from build123d import *

# Parameters (mm, degrees)
F0_R      = 38.1
F1_DEPTH  = 30.48
F2_W      = 45.819147911
F2_H      = 7.0118308067
F3_DEPTH  = 2.54
F4_T      = -2.54
F8_DEPTH  = 9.906
F10_DEPTH = 5.08


with BuildPart() as f1:
    # F0 (on Top) → F1 (new body)
    with BuildSketch(Plane.XY):
        Circle(F0_R)
    extrude(amount=F1_DEPTH)

    # F2 (on face) → F3 (join)
    with BuildSketch(Plane.XY.offset(30.48)):
        with Locations((0.8893240733, -19.5669056848)):
            Rectangle(F2_W, F2_H)
    extrude(amount=F3_DEPTH)

    # F4 (hollow: no face is removed)
    offset(amount=F4_T, kind=Kind.INTERSECTION, mode=Mode.SUBTRACT)

    # F7 (on face) → F8 (cut)
    with BuildSketch(Plane.XY.offset(30.48)):
        Polygon((-15.4119321378, -12.1194338849), (-14.841485885, -15.7707315361), (5.0025711535, -15.7707315361), (6.1164895305, -14.8400934836), (6.1164895305, -11.340892916), (6.3189007342, -9.2710563913), (6.0210963711, -6.8141715601), (6.0048130108, -5.5709355934), (5.6325580226, -4.6775222713), (6.0792639852, -3.5607567247), (6.0792639852, -2.0221695727), (5.7286338997, -1.0273779467), (9.9040070724, 0.4442985472), (11.7219447857, 2.5462731296), (11.7219447857, 4.9659329975), (15.7423027558, 7.0877885023), (22.1039241878, 10.3067904288), (25.4188793848, 10.3067904288), (29.9926726737, 12.4215105659), (30.7439389297, 15.0509480497), (29.6866364668, 17.4833167877), (25.6525882866, 18.8981650481), (18.5155458163, 17.708657504), (16.6474783241, 16.844945549), (9.1134678884, 13.3615516624), (7.5662216179, 11.7286253879), (1.8378060551, 10.445210726), (1.149144816, 10.8521465371), (3.3716449027, 11.5721119727), (5.3750247236, 13.2937669913), (5.9697784957, 15.1093309904), (5.5432569709, 17.361162805), (5.2361546324, 17.7185181528), (2.1184887737, 17.7185181528), (1.3361625606, 21.336780861), (1.3361625606, 23.9771343768), (0, 26.2263249606), (0, 27.1613527107), (-3.5394631901, 30.5318216514), (-5.2709043957, 31.7105762661), (-8.7543707341, 32.132551074), (-11.3128684461, 31.4410664141), (-14.5628526807, 30.542133376), (-16.7756080627, 28.8825668395), (-19.0620572539, 25.78573856), (-20.3636531951, 22.1986565316), (-20.7315385342, 18.6494737864), (-19.479425624, 13.39059975), (-15.4119321378, 10.9802337791), (-19.0177896293, 7.0877885023), (-19.0177896293, 0.4442985472), (-15.4119321378, -3.7730513141), (-16.0732436925, -8.2028741017), align=None)
    extrude(amount=-F8_DEPTH, mode=Mode.SUBTRACT)

    # F9 (on face) → F10 (join)
    with BuildSketch(Plane.XY.offset(30.48)):
        Polygon((9.2707704753, 15.7535430044), (10.2326864312, 16.7216230184), (-7.1297219356, 16.7216230184), (-13.6908106506, 14.8423165083), (-17.4043960869, 9.4877332449), (-19.9085921049, 6.8410946988), (-19.9085921049, 1.7150167664), (-19.6581706405, -3.6766524427), (-15.2726136148, -5.7415137999), (-13.1471836939, -2.1741164383), (-7.5955540778, 6.8410946988), (4.2351128765, 10.4722213), (9.2707704753, 14.7913218218), align=None)
        Polygon((3.8815487642, 1.0813763365), (6.6431248561, 0.6791502237), (9.9622569978, 2.7536081616), (11.7555428296, 4.9633402377), (15.3087614144, 6.8410946988), (21.8024684188, 8.8341752525), (30.4993893951, 12.0195187628), (30.8451298624, 16.7216230184), (27.3877009749, 19.3492695689), (19.6581706405, 19.6126438677), (12.7007676991, 15.7535430044), (10.8933802694, 14.2285590991), (9.2707704753, 12.8604179814), (2.2486662492, 8.0840246186), (1.4972069766, 4.3447160861), align=None)
    extrude(amount=F10_DEPTH)


solid = f1.part
The model under review builds one solid part; all positions refer to its coordinate system, in mm. A direction names the side the tool comes from. Round coordinates to 2 decimals unless told otherwise and drop trailing zeros. Write each loop counter-clockwise with the first axis right and the second up, starting at its lowest first coordinate (ties: lowest second). Pieces come first, ordered by that corner, then holes. Notation, with made-up numbers: (-15, 37) - (36, 37) arc R33 ccw to (36, 69) - close; hole circle Ø5 at (31.25, 54.5). An arc over 180 degrees is marked (long way). One line per item, written item: value. Start each with the question number.
1. The part is to be moulded in two halves that separate along Y. For faces 5 (the face through (1, -23.073, 32)), 6 (the face through (-15.522, 12.203, 32.984)), 7 (the face through (2.7, 2.7, 33)), say which applies: released by +Y, released by -Y, zero draft, split by the parting line, or undercut.
2. Machinability: for faces 1 (the face through (10.846, 3.843, 32.984)), 2 (the face through (-22.02, -20, 32)), 3 (the face through (-4.39, 31.11, 29.23)), 4 (the face through (2.245, 11.207, 29.228)), which of the approach directions +Z, -Z, +X, -X, +Y, -Y give a long, thin tool a straight path to every point of the face, cutting with its end or side? Answer none if there is none.
3. Clearance check with flat-ended pins moving along their axes: P1, Ø2, axis at y = -19, z = 26.5, coming from the +X side; P2, Ø8, axis at x = 24.5, z = 19.5, coming from the +Y side; P3, Ø0.7, axis at y = 4, z = 29, coming from the -X side. State where each tip first meets the part, or that it passes through.
4. Consider section A-A on z = 25.5. Write out the cut boundary in (x, y).
5. To check wall thickness, follow L1, parallel to Z at x = -7, y = -16; L2, parallel to Y at x = 0, z = 9; L3, parallel to Z at x = 12.5, y = -20. State the ranges of each line that lie inside material, in increasing order. Write a range as from..to.
Checks:
1. face 5: released by -Y
1. face 6: released by +Y
1. face 7: undercut
2. face 1: +Z, +X
2. face 2: +Z, -X, +Y, -Y
2. face 3: +Z
2. face 4: none
3. P1: stops at x = 33.58
3. P2: stops at y = 32.11
3. P3: stops at x = -37.92
4. outline: circle Ø76.2 at (0, 0); hole circle Ø71.12 at (0, 0)
5. L1: z = 0..2.54, 27.94..30.48
5. L2: y = -38.1..-35.56, 35.56..38.1
5. L3: z = 0..2.54, 30.48..33.02
